Check sheet for the modelled part. Datum: model origin and axes. Units: mm. Face numbers are marked on the shaded views. A direction names the side the tool comes from. Give positions to 0.01 mm unless a question says otherwise; leave off trailing zeros. Write each loop counter-clockwise with the first axis right and the second up, starting at its lowest first coordinate (ties: lowest second). Pieces come first, ordered by that corner, then holes. Notation, with made-up numbers: M 88.5,89 L 111.5,89 A26 ccw 111.5,115 Z; hole C 63,-13 d4. An arc over 180 degrees is marked long. Write item = value, one per line. Start each with the question number.
1) Sectioned sample at B-B, the plane x = 7.25. Record the cut outline in (y, z).
2) Draft check along Y on the marked faces 3, 4 and 5. Enter one of: pulls with the +Y half, pulls with the -Y half, needs draft (parallel to the pull), parting line crosses it, or undercut.
3) Gauge pin test, flat ends, axial feed: pin 1 (3 mm diameter, centred on y = 50.5, z = 1.5, fed in from -X); pin 2 (1 mm diameter, centred on x = -6, y = 112, fed in from +Z); pin 3 (1.5 mm diameter, centred on y = 77, z = -7, fed in from -X); pin 4 (3.5 mm diameter, centred on y = 65.5, z = -2.5, fed in from +X). Record the tip position at first contact, or that the pin passes through.
4) Set-up check for the marked faces 1 and 2: record each of +Z, -Z, +X, -X, +Y, -Y from which the full face is reachable in a straight line by a thin tool's end or side.
5) Scan lines: L1, parallel to Y at x = -4.25, z = 0.5; L2, parallel to Z at x = -1.5, y = 118; L3, parallel to Y at x = 0, z = 0. Record each from-to range of solid material in increasing order.
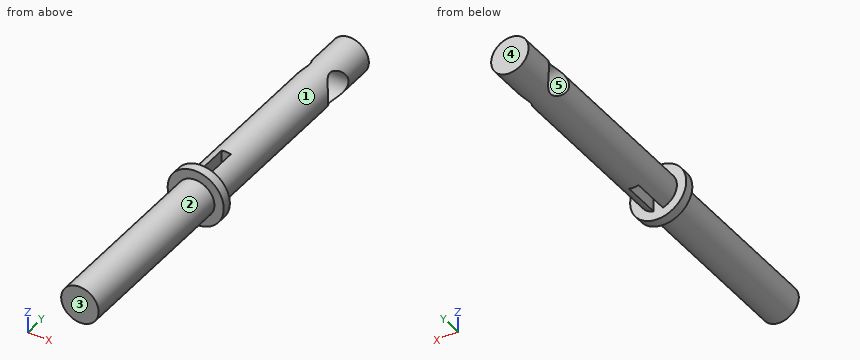
from build123d import *

# Parameters (mm, degrees)
SKETCH1_R           = 6
BOSS_EXTRUDE1_DEPTH = 100
SKETCH2_W           = 3
SKETCH2_H           = 12
CUT_EXTRUDE2_DEPTH  = 50
SKETCH3_R           = 2.5
CUT_EXTRUDE3_DEPTH  = 50
BOSS_EXTRUDE2_START = -60
SKETCH4_R           = 9
BOSS_EXTRUDE2_DEPTH = 3
SKETCH5_R           = 6
BOSS_EXTRUDE3_DEPTH = 10
SKETCH6_R           = 2.5
CUT_EXTRUDE4_DEPTH  = 10
SKETCH7_R           = 6
CUT_EXTRUDE5_DEPTH  = 12
SKETCH8_R           = 6
BOSS_EXTRUDE4_DEPTH = 30
SKETCH10_R          = 5
CUT_EXTRUDE6_DEPTH  = 30
BOSS_EXTRUDE5_START = -40
SKETCH11_R          = 6
BOSS_EXTRUDE5_DEPTH = 40
SKETCH12_R          = 6
BOSS_EXTRUDE6_DEPTH = 5
SKETCH13_R          = 5
CUT_EXTRUDE7_DEPTH  = 27.5


with BuildPart() as part:
    # Sketch1 → Boss-Extrude1 (new body)
    with BuildSketch(Plane(origin=(0, 0, 0), x_dir=(1, 0, 0), z_dir=(0, 1, 0))):
        with Locations(Location((0, 0, 0), (0, 0, 270))):
            Circle(SKETCH1_R)
    extrude(amount=BOSS_EXTRUDE1_DEPTH)

    # Sketch2 → Cut-Extrude2 (cut, symmetric)
    with BuildSketch(Plane.XY):
        with Locations((0, 66)):
            Rectangle(SKETCH2_W, SKETCH2_H)
    extrude(amount=CUT_EXTRUDE2_DEPTH, both=True, mode=Mode.SUBTRACT)

    # Sketch3 → Cut-Extrude3 (cut, symmetric)
    with BuildSketch(Plane.XY):
        with Locations(Location((0, 95, 0), (0, 0, 90))):
            Circle(SKETCH3_R)
    extrude(amount=CUT_EXTRUDE3_DEPTH, both=True, mode=Mode.SUBTRACT)

    # Sketch4 → Boss-Extrude2 (add)
    with BuildSketch(Plane.XZ.offset(BOSS_EXTRUDE2_START)):
        with Locations(Location((0, 0, 0), (0, 0, 270))):
            Circle(SKETCH4_R)
    extrude(amount=BOSS_EXTRUDE2_DEPTH)

    # Sketch5 → Boss-Extrude3 (add, symmetric)
    with BuildSketch(Plane(origin=(0, 100, 0), x_dir=(1, 0, 0), z_dir=(0, 1, 0))):
        with Locations(Location((0, 0, 0), (0, 0, 90))):
            Circle(SKETCH5_R)
    extrude(amount=BOSS_EXTRUDE3_DEPTH, both=True)

    # Sketch6 → Cut-Extrude4 (cut, symmetric)
    with BuildSketch(Plane.XY):
        with Locations((0, 105)):
            Circle(SKETCH6_R)
    extrude(amount=CUT_EXTRUDE4_DEPTH, both=True, mode=Mode.SUBTRACT)

    # Sketch7 → Cut-Extrude5 (cut)
    with BuildSketch(Plane(origin=(0, 110, 0), x_dir=(1, 0, 0), z_dir=(0, 1, 0))):
        with Locations(Location((0, 0, 0), (0, 0, 75.522487814))):
            Circle(SKETCH7_R)
    extrude(amount=-CUT_EXTRUDE5_DEPTH, mode=Mode.SUBTRACT)

    # Sketch8 → Boss-Extrude4 (add)
    with BuildSketch(Plane(origin=(0, 98, 0), x_dir=(1, 0, 0), z_dir=(0, 1, 0))):
        with Locations(Location((0, 0, 0), (0, 0, 75.522487814))):
            Circle(SKETCH8_R)
    extrude(amount=BOSS_EXTRUDE4_DEPTH)

    # Sketch10 → Cut-Extrude6 (cut, symmetric)
    with BuildSketch(Plane.XY):
        with Locations((0, 113)):
            Circle(SKETCH10_R)
    extrude(amount=CUT_EXTRUDE6_DEPTH, both=True, mode=Mode.SUBTRACT)

    # Sketch11 → Boss-Extrude5 (add)
    with BuildSketch(Plane(origin=(0, 128, 0), x_dir=(1, 0, 0), z_dir=(0, 1, 0)).offset(BOSS_EXTRUDE5_START)):
        with Locations(Location((0, 0, 0), (0, 0, 75.522487814))):
            Circle(SKETCH11_R)
    extrude(amount=BOSS_EXTRUDE5_DEPTH)

    # Sketch12 → Boss-Extrude6 (add)
    with BuildSketch(Plane(origin=(0, 128, 0), x_dir=(1, 0, 0), z_dir=(0, 1, 0))):
        with Locations(Location((0, 0, 0), (0, 0, 75.522487814))):
            Circle(SKETCH12_R)
    extrude(amount=BOSS_EXTRUDE6_DEPTH)

    # Sketch13 → Cut-Extrude7 (cut, symmetric)
    with BuildSketch(Plane(origin=(0, 0, 0), x_dir=(0, 0, -1), z_dir=(1, 0, 0))):
        with Locations((0, 118)):
            Circle(SKETCH13_R)
    extrude(amount=CUT_EXTRUDE7_DEPTH, both=True, mode=Mode.SUBTRACT)


solid = part.part
Data:
q1.outline = M 57,-5.33 L 60,-5.33 L 60,5.33 L 57,5.33 Z
q2.face_3 = pulls with the -Y half
q2.face_4 = pulls with the +Y half
q2.face_5 = undercut
q3.pin_1 = -6
q3.pin_2 = 2.4
q3.pin_3 = through
q3.pin_4 = 5.95
q4.face_1 = +Y
q4.face_2 = -Y
q5.L1 = 0 to 113.03, 122.97 to 133
q5.L2 = -5.81 to -5, 5 to 5.81
q5.L3 = 0 to 60, 72 to 113, 123 to 133
